Part model, mm, in its own coordinate system. Face numbers are marked on the shaded views. A direction names the side the tool comes from. Give positions to 0.01 mm unless a question says otherwise; leave off trailing zeros. Loops run counter-clockwise (first coordinate to the right, second up) from the corner with the lowest first, then second, coordinate; pieces in that order, holes last. Notation, with made-up numbers: (64.25, 12.25) -> (98.25, 12.25) arc R21 cw to (98.25, 47.25) -> close; hole circle Ø1 at (55, 27). An arc over 180 degrees is marked (long way). One line per question, with ' | ' between items.
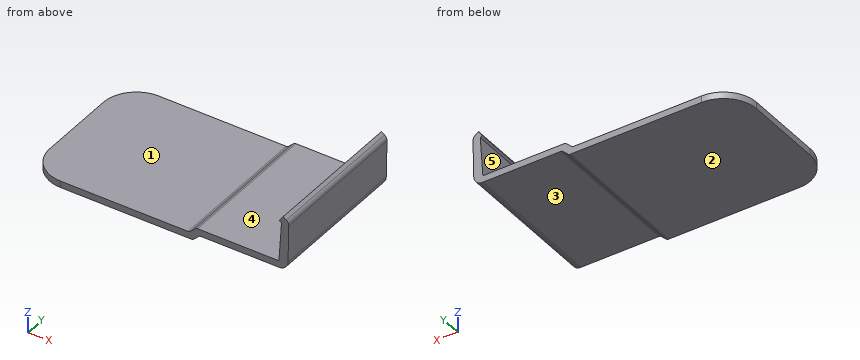
```python
from build123d import *

# Parameters (mm, degrees)
F1_DEPTH = 22
F3_DEPTH = 2


with BuildPart() as f1:
    # F0 (on Front) → F1 (new body, symmetric)
    with BuildSketch(Plane.XZ):
        with BuildLine():
            Line((-40, 0), (-0.4058661959, 0))
            ThreePointArc((-0.4058661959, 0), (-0.0297944203, 0.073409465), (0.2910628996, 0.2828599608))
            Line((0.2910628996, 0.2828599608), (1.7669371004, 1.7171400392))
            ThreePointArc((1.7669371004, 1.7171400392), (2.0877944203, 1.926590535), (2.4638661959, 2))
            Line((2.4638661959, 2), (26.037, 2))
            ThreePointArc((26.037, 2), (27.9687843496, 2.7891547709), (28.7954749436, 4.705176349))
            Line((28.7954749436, 4.705176349), (29.016465998, 16.0310205539))
            ThreePointArc((29.016465998, 16.0310205539), (28.8276722638, 16.8546583092), (28.2736767263, 17.4927109486))
            Line((28.2736767263, 17.4927109486), (27.3333525812, 18.1512658075))
            Line((27.3333525812, 18.1512658075), (26.1860444646, 16.5130704329))
            Line((26.1860444646, 16.5130704329), (26.8254471929, 16.0652655182))
            Line((26.8254471929, 16.0652655182), (26.037, 4))
            Line((26.037, 4), (1.4428661959, 4))
            ThreePointArc((1.4428661959, 4), (1.0667944203, 3.926590535), (0.7459371004, 3.7171400392))
            Line((0.7459371004, 3.7171400392), (-0.7299371004, 2.2828599608))
            ThreePointArc((-0.7299371004, 2.2828599608), (-1.0507944203, 2.073409465), (-1.4268661959, 2))
            Line((-1.4268661959, 2), (-40, 2))
            Line((-40, 2), (-40, 0))
        make_face()
    extrude(amount=F1_DEPTH, both=True)

    # F2 (on face) → F3 (join)
    with BuildSketch(Plane.XY.offset(2)):
        with BuildLine():
            Line((-50, 12), (-50, -12))
            ThreePointArc((-50, -12), (-47.0710678119, -19.0710678119), (-40, -22))
            Line((-40, -22), (-40, 22))
            ThreePointArc((-40, 22), (-47.0710678119, 19.0710678119), (-50, 12))
        make_face()
    extrude(amount=-F3_DEPTH)


solid = f1.part
```
1) Saw through at B-B (x = -6). Give the cut face in (y, z), and give its area (3 significant figures).
Found:
outline: (-22, 0) -> (22, 0) -> (22, 2) -> (-22, 2) -> close | area: 88.0 mm2
2) Pull direction Z, two halves, no side cores. Call the marked faces 3, 4 and 5: pulls with the +Z half, pulls with the -Z half, needs draft (parallel to the pull), parting line crosses it, or undercut.
Found:
face 3: pulls with the -Z half | face 4: pulls with the +Z half | face 5: undercut
3) Saw through at D-D (y = -17). Give the cut face in (x, z), and give its area (3 significant figures).
Found:
outline: (-48.66, 0) -> (-0.41, 0) arc R1 ccw to (0.29, 0.28) -> (1.77, 1.72) arc R1 cw to (2.46, 2) -> (26.04, 2) arc R2.76 ccw to (28.8, 4.71) -> (29.02, 16.03) arc R1.74 ccw to (28.27, 17.49) -> (27.33, 18.15) -> (26.19, 16.51) -> (26.83, 16.07) -> (26.04, 4) -> (1.44, 4) arc R1 ccw to (0.75, 3.72) -> (-0.73, 2.28) arc R1 cw to (-1.43, 2) -> (-48.66, 2) -> close | area: 189 mm2
4) Drill centre lines: line 1 (Z direction, x = 9, y = -16.5); line 2 (Z direction, x = -26.5, y = -20); line 3 (X direction, y = -17.5, z = 6.25). Where is each one in solid material? Low to high.
Found:
line 1: 2 to 4 | line 2: 0 to 2 | line 3: 26.18 to 28.83
5) Saw through at C-C (z = 7.25). Give the cut face in (x, y), and give its area (3 significant figures).
Found:
outline: (26.25, -22) -> (28.85, -22) -> (28.85, 22) -> (26.25, 22) -> close | area: 114 mm2
6) Saw through at A-A (y = -8.5). Give the cut face in (x, z), and give its area (3 significant figures).
Found:
outline: (-50, 0) -> (-0.41, 0) arc R1 ccw to (0.29, 0.28) -> (1.77, 1.72) arc R1 cw to (2.46, 2) -> (26.04, 2) arc R2.76 ccw to (28.8, 4.71) -> (29.02, 16.03) arc R1.74 ccw to (28.27, 17.49) -> (27.33, 18.15) -> (26.19, 16.51) -> (26.83, 16.07) -> (26.04, 4) -> (1.44, 4) arc R1 ccw to (0.75, 3.72) -> (-0.73, 2.28) arc R1 cw to (-1.43, 2) -> (-50, 2) -> close | area: 191 mm2
7) Tool access for the marked faces 1 and 2: list every direction of +Z, -Z, +X, -X, +Y, -Y with a clear straight run to the whole face (end or side of a thin tool).
Found:
face 1: +Z, -X, +Y, -Y | face 2: -Z, +X, -X, +Y, -Y
8) Pin check, flat tips, straight feed: P1, Ø5, axis at y = 11, z = 5.5, coming from the +X side; P2, Ø7.5, axis at x = 18.5, y = 10.5, coming from the +Z side; P3, Ø3, axis at x = -40.5, y = -3.5, coming from the +Z side. Stop position of each tip, or through.
Found:
P1: x = 28.86 | P2: z = 4 | P3: z = 2
